Here's how the part is built. I have some questions about the finished solid (model axes, mm). Face numbers are marked on the shaded views. A direction names the side the tool comes from. Coordinates: 2 decimals unless noted, no trailing zeros. Loops run counter-clockwise (first coordinate to the right, second up) from the corner with the lowest first, then second, coordinate; pieces in that order, holes last. Notation, with made-up numbers: (5, 71) -> (18, 71) arc R27 cw to (18, 99) -> close; hole circle Ø10 at (-21, -32.5). An arc over 180 degrees is marked (long way). Answer as a JSON object with one key per item and string values. Group by question number.
Q1. I want a section at D-D on x = -24. Write out the boundary of the cut face in (y, z).
Q2. I want a section at A-A on y = 0. Count the separate pieces of the cut face and the enclosed holes in it, then the cut area to 3 significant figures.
Q3. I'm going to push flat-ended pins straight in: pin 1 (6 mm diameter, centred on x = 18.5, z = 8, fed in from +Y); pin 2 (4 mm diameter, centred on y = -10.5, z = 4, fed in from +X); pin 3 (9 mm diameter, centred on x = 0, y = 0, fed in from -Z); pin 4 (1 mm diameter, centred on x = 15, y = 8, fed in from -Z). Where does each tip first touch, or does it pass through?
Q4. I want a section at C-C on z = -0.75. Write out the boundary of the cut face in (x, y), then the cut area to 3 significant figures.
Q5. I want a section at B-B on x = -10. Write out the boundary of the cut face in (y, z), then the cut area to 3 significant figures.
Q6. On a 3-axis mill with a long thin cutter (end or side, diameter ignored), from which of +Z, -Z, +X, -X, +Y, -Y can I reach the whole of each face in a straight line? I mean the marked faces 1, 2 and 3. Say none if no direction works.
Q7. I need wall thicknesses on line 1 (Y direction, x = -16, z = 12.9); line 2 (X direction, y = 11.5, z = 5); line 3 (X direction, y = 0, z = 7.25). Which ranges of each line are inside material? Lowest first, please.
Q8. Thinking about a two-plate mould opening in Y: for the marked faces 4, 5, 6 and 7, which applies, released by +Y, released by -Y, zero draft, split by the parting line, or undercut?
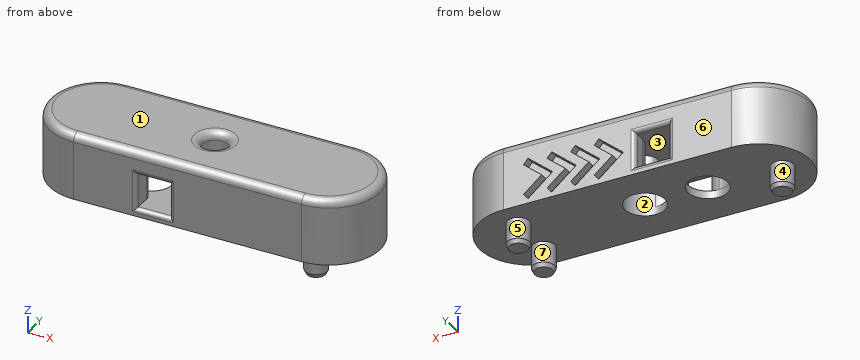
```python
from build123d import *
from OCP.BRepFilletAPI import BRepFilletAPI_MakeChamfer

# Parameters (mm, degrees)
SKETCH1_R             = 2.8
BOSS_EXTRUDE1_DEPTH   = 6.4
BOSS_EXTRUDE1_2_DEPTH = 6.4
BOSS_EXTRUDE1_3_DEPTH = 6.4
SKETCH1_3_R           = 5.05
BOSS_EXTRUDE2_DEPTH   = 2
BOSS_EXTRUDE3_DEPTH   = 8.8
SKETCH6_R             = 5.05
SKETCH6_R_2           = 3.25
BOSS_EXTRUDE4_DEPTH   = 6
SKETCH6_4_R           = 5.05
CUT_EXTRUDE1_DEPTH    = 4
FILLET1_R             = 2
FILLET2_R             = 1
CHAMFER1_SIZE         = 0.5
CHAMFER1_SIZE2        = 1
CUT_EXTRUDE2_DEPTH    = 2


with BuildPart() as part:
    # Sketch1 → Boss-Extrude1 (new body)
    with BuildSketch(Plane.XY):
        with Locations((29, 6)):
            Circle(SKETCH1_R)
    extrude(amount=-BOSS_EXTRUDE1_DEPTH)



with BuildPart() as body_2:
    # Sketch1 → Boss-Extrude1 2 (new body)
    with BuildSketch(Plane.XY):
        with Locations((29, -6)):
            Circle(SKETCH1_R)
    extrude(amount=-BOSS_EXTRUDE1_2_DEPTH)


with BuildPart() as body_3:
    # Sketch1 → Boss-Extrude1 3 (new body)
    with BuildSketch(Plane.XY):
        with Locations((-35, 0)):
            Circle(SKETCH1_R)
    extrude(amount=-BOSS_EXTRUDE1_3_DEPTH)


with BuildPart() as part_1:
    add(part.part)

    add(body_2.part)  # Boss-Extrude2 merges body 2

    add(body_3.part)  # Boss-Extrude2 merges body 3
    # Sketch1<3> → Boss-Extrude2 (add)
    with BuildSketch(Plane.XY):
        with BuildLine():
            Line((29, 13), (-29, 13))
            ThreePointArc((-29, 13), (-42, 0), (-29, -13))
            Line((-29, -13), (29, -13))
            ThreePointArc((29, -13), (42, 0), (29, 13))
        make_face()
        with Locations((-16, 0)):
            Circle(SKETCH1_3_R, mode=Mode.SUBTRACT)
        Circle(SKETCH1_3_R, mode=Mode.SUBTRACT)
    extrude(amount=BOSS_EXTRUDE2_DEPTH)

    # Sketch5 → Boss-Extrude3 (add)
    with BuildSketch(Plane.XY.offset(2)):
        with BuildLine():
            Line((-4.5, -9.55), (-4.5, -13))
            Line((-4.5, -13), (29, -13))
            ThreePointArc((29, -13), (42, 0), (29, 13))
            Line((29, 13), (-4.5, 13))
            Line((-4.5, 13), (-4.5, 9.55))
            ThreePointArc((-4.5, 9.55), (-3.181980515, 6.368019485), (0, 5.05))
            ThreePointArc((0, 5.05), (5.05, 0), (0, -5.05))
            ThreePointArc((0, -5.05), (-3.181980515, -6.368019485), (-4.5, -9.55))
        make_face()
        with BuildLine():
            Line((-13, 8.25), (-13, 13))
            Line((-13, 13), (-29, 13))
            ThreePointArc((-29, 13), (-42, 0), (-29, -13))
            Line((-29, -13), (-13, -13))
            Line((-13, -13), (-13, -8.25))
            ThreePointArc((-13, -8.25), (-13.878679656, -6.128679656), (-16, -5.25))
            ThreePointArc((-16, -5.25), (-21.25, 0), (-16, 5.25))
            ThreePointArc((-16, 5.25), (-13.878679656, 6.128679656), (-13, 8.25))
        make_face()
    extrude(amount=BOSS_EXTRUDE3_DEPTH)

    # Sketch6 → Boss-Extrude4 (add)
    # profile 1 of 3: a face of its own
    with BuildSketch(Plane.XY.offset(10.8)):
        with BuildLine():
            ThreePointArc((-16, -5.25), (-21.25, 0), (-16, 5.25))
            ThreePointArc((-16, 5.25), (-13.878679656, 6.128679656), (-13, 8.25))
            Line((-13, 8.25), (-13, 13))
            Line((-13, 13), (-29, 13))
            ThreePointArc((-29, 13), (-42, 0), (-29, -13))
            Line((-29, -13), (-13, -13))
            Line((-13, -13), (-13, -8.25))
            ThreePointArc((-13, -8.25), (-13.878679656, -6.128679656), (-16, -5.25))
        make_face()
    # profile 2 of 3: a face of its own
    with BuildSketch(Plane.XY.offset(10.8)):
        with BuildLine():
            ThreePointArc((29, -13), (42, 0), (29, 13))
            Line((29, 13), (-13, 13))
            Line((-13, 13), (-13, 8.25))
            ThreePointArc((-13, 8.25), (-13.878679656, 6.128679656), (-16, 5.25))
            ThreePointArc((-16, 5.25), (-21.25, 0), (-16, -5.25))
            ThreePointArc((-16, -5.25), (-13.878679656, -6.128679656), (-13, -8.25))
            Line((-13, -8.25), (-13, -13))
            Line((-13, -13), (29, -13))
        make_face()
        with Locations((-16, 0)):
            Circle(SKETCH6_R, mode=Mode.SUBTRACT)
        Circle(SKETCH6_R_2, mode=Mode.SUBTRACT)
    # profile 3 of 3: a face of its own
    with BuildSketch(Plane.XY.offset(10.8)):
        with Locations((-16, 0)):
            Circle(SKETCH6_R)
    extrude(amount=BOSS_EXTRUDE4_DEPTH)

    # Sketch6<4> → Cut-Extrude1 (cut)
    with BuildSketch(Plane.XY.offset(10.8)):
        with Locations((-16, 0)):
            Circle(SKETCH6_4_R)
    extrude(amount=CUT_EXTRUDE1_DEPTH, mode=Mode.SUBTRACT)

    # Fillet1
    fillet1_edges = [part_1.edges().sort_by_distance(p)[0] for p in [
        (-3.25, 0, 16.8),
        (42, 0, 16.8),
        (0, 13, 16.8),
        (-42, 0, 16.8),
        (0, -13, 16.8),
    ]]
    fillet(fillet1_edges, radius=FILLET1_R)

    # Fillet2
    fillet2_edges = [part_1.edges().sort_by_distance(p)[0] for p in [
        (-8.75, 13, 2),
        (-4.5, 13, 6.4),
        (-4.5, -13, 6.4),
        (-8.75, -13, 2),
        (-13, -13, 6.4),
        (-13, 13, 6.4),
        (-8.75, 13, 10.8),
        (-8.75, -13, 10.8),
    ]]
    fillet(fillet2_edges, radius=FILLET2_R)

    # Chamfer1: one chamfer whose edges measure the first distance from different faces: ONE call of the kernel's chamfer builder (chamfer() names one face for all edges)
    chamfer1_edges_1 = [part_1.edges().sort_by_distance(p)[0] for p in [
        (26.2, 6, -6.4),
    ]]
    chamfer1_side_1 = [part_1.faces().sort_by_distance(p)[0] for p in [
        (29, 6, -6.4),
    ]]
    chamfer1_edges_2 = [part_1.edges().sort_by_distance(p)[0] for p in [
        (26.2, -6, -6.4),
    ]]
    chamfer1_side_2 = [part_1.faces().sort_by_distance(p)[0] for p in [
        (29, -6, -6.4),
    ]]
    chamfer1_edges_3 = [part_1.edges().sort_by_distance(p)[0] for p in [
        (-37.8, 0, -6.4),
    ]]
    chamfer1_side_3 = [part_1.faces().sort_by_distance(p)[0] for p in [
        (-35, 0, -6.4),
    ]]
    chamfer1 = BRepFilletAPI_MakeChamfer(part_1.part.solid().wrapped)
    for e in chamfer1_edges_1:
        chamfer1.Add(CHAMFER1_SIZE, CHAMFER1_SIZE2, e.wrapped, chamfer1_side_1[0].wrapped)  # the first distance lies on this face
    for e in chamfer1_edges_2:
        chamfer1.Add(CHAMFER1_SIZE, CHAMFER1_SIZE2, e.wrapped, chamfer1_side_2[0].wrapped)  # the first distance lies on this face
    for e in chamfer1_edges_3:
        chamfer1.Add(CHAMFER1_SIZE, CHAMFER1_SIZE2, e.wrapped, chamfer1_side_3[0].wrapped)  # the first distance lies on this face
    add(Compound.cast(chamfer1.Shape()), mode=Mode.REPLACE)

    # Sketch7 → Cut-Extrude2 (cut)
    with BuildSketch(Plane(origin=(0, 13, 0), x_dir=(1, 0, 0), z_dir=(0, 1, 0))):
        Polygon((-1.5, -6.4), (4.73955185, -11.635605656), (5.896569547, -10.256725658), (1.300302888, -6.4), (5.896569547, -2.543274342), (4.73955185, -1.164394344), align=None)
        Polygon((10.73955185, -1.164394344), (4.5, -6.4), (10.73955185, -11.635605656), (11.896569547, -10.256725658), (7.300302888, -6.4), (11.896569547, -2.543274342), align=None)
        Polygon((16.73955185, -1.164394344), (10.5, -6.4), (16.73955185, -11.635605656), (17.896569547, -10.256725658), (13.300302888, -6.4), (17.896569547, -2.543274342), align=None)
        Polygon((22.73955185, -1.164394344), (16.5, -6.4), (22.73955185, -11.635605656), (23.896569547, -10.256725658), (19.300302888, -6.4), (23.896569547, -2.543274342), align=None)
    extrude(amount=-CUT_EXTRUDE2_DEPTH, mode=Mode.SUBTRACT)


solid = part_1.part
```
Result set:
{
 "1": {"outline": "(-13, 0) -> (13, 0) -> (13, 14.8) arc R2 ccw to (11, 16.8) -> (-11, 16.8) arc R2 ccw to (-13, 14.8) -> close"},
 "2": {"separate pieces": "3", "enclosed holes": "0", "area": "1,090 mm²"},
 "3": {"pin 1": "stops at y = 13", "pin 2": "stops at x = 38.84", "pin 3": "stops at z = 10.8", "pin 4": "stops at z = 0"},
 "4": {"outline": "circle Ø5.6 at (-35, 0); circle Ø5.6 at (29, -6); circle Ø5.6 at (29, 6)", "area": "73.9 mm²"},
 "5": {"outline": "(-13, 0) -> (13, 0) -> (13, 1) arc R1 ccw to (12, 2) -> (-12, 2) arc R1 ccw to (-13, 1) -> close; (-13, 11.8) arc R1 ccw to (-12, 10.8) -> (12, 10.8) arc R1 ccw to (13, 11.8) -> (13, 14.8) arc R2 ccw to (11, 16.8) -> (-11, 16.8) arc R2 ccw to (-13, 14.8) -> close", "area": "205 mm²"},
 "6": {"face 1": "+Z, +X, -X, +Y, -Y", "face 2": "-Z", "face 3": "none"},
 "7": {"line 1": "y = -13 to -5.05, 5.05 to 13", "line 2": "x = -35.06 to -13, -4.5 to 0.17, 2.97 to 6.17, 8.97 to 12.17, 14.97 to 18.17, 20.97 to 35.06", "line 3": "x = -42 to -21.25, 5.05 to 42"},
 "8": {"face 4": "split by the parting line", "face 5": "undercut", "face 6": "released by +Y", "face 7": "undercut"}
}
